from build123d import *

# Parameters (mm, degrees)
BOSS_EXTRUDE2_DEPTH = 5
CUT_EXTRUDE1_DEPTH  = 3.7


with BuildPart() as part:
    # Sketch2 → Boss-Extrude2 (new body)
    with BuildSketch(Plane(origin=(0, 0, 0), x_dir=(1, 0, 0), z_dir=(0, 1, 0))):
        Polygon((-7, -7), (-7, 7), (-9.345690752, 9.345690752), (-9.345690752, -9.345690752), align=None)
        Polygon((-7, 7), (-2.5, 7), (-2.5, 8.5), (2.5, 8.5), (2.5, 7), (7, 7), (9.345690752, 9.345690752), (-9.345690752, 9.345690752), align=None)
        Polygon((-2.5, 7), (0, 7), (2.5, 7), (2.5, 8.5), (-2.5, 8.5), align=None)
        Polygon((9.345690752, -9.345690752), (9.345690752, 9.345690752), (7, 7), (7, -7), align=None)
        Polygon((7, -7), (2.5, -7), (2.5, -8.5), (-2.5, -8.5), (-2.5, -7), (-7, -7), (-9.345690752, -9.345690752), (9.345690752, -9.345690752), align=None)
        Polygon((2.5, -7), (0, -7), (-2.5, -7), (-2.5, -8.5), (2.5, -8.5), align=None)
    extrude(amount=BOSS_EXTRUDE2_DEPTH)

    # Sketch3 → Cut-Extrude1 (cut)
    with BuildSketch(Plane.XZ):
        Polygon((2.5, -7), (0, -7), (-2.5, -7), (-2.5, -8.5), (2.5, -8.5), align=None)
        Polygon((-2.5, 7), (0, 7), (2.5, 7), (2.5, 8.5), (-2.5, 8.5), align=None)
    extrude(amount=-CUT_EXTRUDE1_DEPTH, mode=Mode.SUBTRACT)


solid = part.part
Design review of the part built by this model. Coordinates are the model's own, in mm. A direction names the side the tool comes from. Round coordinates to 2 decimals unless told otherwise and drop trailing zeros. Write each loop counter-clockwise with the first axis right and the second up, starting at its lowest first coordinate (ties: lowest second). Pieces come first, ordered by that corner, then holes. Notation, with made-up numbers: (0, -22) - (44, -22) arc R36 cw to (44, 13) - close; hole circle Ø2 at (88.25, 78.25). An arc over 180 degrees is marked (long way). Return JSON: item names as keys, results as strings. Group by question number.
Item 1: We need section A-A on z = -0.5. Write out the cut boundary in (x, y), and give its area (3 significant figures).
Item 2: We need section D-D on z = -7.5. Write out the cut boundary in (x, y), and give its area (3 significant figures).
Item 3: We need section B-B on x = -3.75. Write out the cut boundary in (y, z), and give its area (3 significant figures).
Item 4: We need section C-C on y = 1.95. Write out the cut boundary in (x, z).
Item 5: Insertion check: P1, Ø10, axis at x = -3.5, z = -2.5, coming from the +Y side; P2, Ø1.2, axis at x = 0, z = -7.5, coming from the -Y side. Each pin has a flat end and moves straight along its axis. Give the tip position at first contact, or say it passes through.
Item 6: Machinability: for faces 1 (the face through (0, 2, -8.5)), 2 (the face through (0, 4, 7)), 3 (the face through (0, 2, 9.346)), which of the approach directions +Z, -Z, +X, -X, +Y, -Y give a long, thin tool a straight path to every point of the face, cutting with its end or side? Answer none if there is none.
Item 7: The part is to be moulded in two halves that separate along X. For faces 4 (the face through (0, 2, 8.5)), 5 (the face through (-8, 0, 1)), 6 (the face through (-9.346, 2, 0)), say which applies: pulls with the +X half, pulls with the -X half, needs draft (parallel to the pull), parting line crosses it, or undercut.
Item 8: For probe 1 along X at (y, z) = (2.2, 0); probe 2 along X at (y, z) = (1.15, 8), list the stretches that pass through material, from the lowest coordinate up. Write a range as [from, to].
Model answer:
{
 "1": {"outline": "(-9.35, 0) - (-7, 0) - (-7, 5) - (-9.35, 5) - close; (7, 0) - (9.35, 0) - (9.35, 5) - (7, 5) - close", "area": "23.5 mm²"},
 "2": {"outline": "(-9.35, 0) - (-2.5, 0) - (-2.5, 3.7) - (2.5, 3.7) - (2.5, 0) - (9.35, 0) - (9.35, 5) - (-9.35, 5) - close", "area": "75.0 mm²"},
 "3": {"outline": "(0, -9.35) - (5, -9.35) - (5, -7) - (0, -7) - close; (0, 7) - (5, 7) - (5, 9.35) - (0, 9.35) - close", "area": "23.5 mm²"},
 "4": {"outline": "(-9.35, -9.35) - (9.35, -9.35) - (9.35, 9.35) - (-9.35, 9.35) - close; hole (-7, -7) - (-2.5, -7) - (-2.5, -8.5) - (2.5, -8.5) - (2.5, -7) - (7, -7) - (7, 7) - (2.5, 7) - (2.5, 8.5) - (-2.5, 8.5) - (-2.5, 7) - (-7, 7) - close"},
 "5": {"P1": "stops at y = 5", "P2": "stops at y = 3.7"},
 "6": {"face 1": "-Y", "face 2": "+Y, -Y", "face 3": "+Z, +X, -X, +Y, -Y"},
 "7": {"face 4": "undercut", "face 5": "needs draft", "face 6": "pulls with the -X half"},
 "8": {"probe 1": "x = [-9.35, -7], [7, 9.35]", "probe 2": "x = [-9.35, -2.5], [2.5, 9.35]"}
}
